Source: CAD feature listing. Evaluate the final solid. Frame: model axes, mm. Give positions to 0.01 mm unless a question says otherwise; leave off trailing zeros. Order: outer loops, then holes, each group sorted by start corner. A loop starts at its lowest first (then second) coordinate and runs counter-clockwise, first axis right, second up.
```python
from build123d import *

# Parameters (mm, degrees)
SKETCH1_R           = 88.9
SKETCH1_R_2         = 2
BOSS_EXTRUDE1_DEPTH = 1.016
SKETCH3_R           = 1.25
SKETCH3_R_2         = 2.25
CUT_EXTRUDE2_DEPTH  = 3.175
SKETCH4_R           = 4.2
CUT_EXTRUDE3_DEPTH  = 10


with BuildPart() as part:
    # Sketch1 → Boss-Extrude1 (new body)
    with BuildSketch(Plane.XY):
        Circle(SKETCH1_R)
        with Locations((41.275, 71.490397082)):
            Circle(SKETCH1_R_2, mode=Mode.SUBTRACT)
        with Locations((82.55, 0)):
            Circle(SKETCH1_R_2, mode=Mode.SUBTRACT)
        with Locations((41.275, -71.490397082)):
            Circle(SKETCH1_R_2, mode=Mode.SUBTRACT)
        with Locations((-41.275, -71.490397082)):
            Circle(SKETCH1_R_2, mode=Mode.SUBTRACT)
        with Locations((-82.55, 0)):
            Circle(SKETCH1_R_2, mode=Mode.SUBTRACT)
        with Locations((-41.275, 71.490397082)):
            Circle(SKETCH1_R_2, mode=Mode.SUBTRACT)
    extrude(amount=BOSS_EXTRUDE1_DEPTH)

    # Sketch3 → Cut-Extrude2 (cut)
    with BuildSketch(Plane.XY.offset(1.016)):
        with Locations((-46.5, 40.2)):
            Circle(SKETCH3_R)
        with Locations((46.5, 40.2)):
            Circle(SKETCH3_R)
        with Locations((46.5, -14.8)):
            Circle(SKETCH3_R)
        with Locations((-46.5, -14.8)):
            Circle(SKETCH3_R)
        with Locations((-31.700000009, 45.8)):
            Circle(SKETCH3_R_2)
    extrude(amount=-CUT_EXTRUDE2_DEPTH, mode=Mode.SUBTRACT)

    # Sketch4 → Cut-Extrude3 (cut)
    with BuildSketch(Plane.XY.offset(1.016)):
        with Locations((60.96, 29.21)):
            Circle(SKETCH4_R)
        with Locations((60.96, 13.97)):
            Circle(SKETCH4_R)
        with Locations((60.96, -1.27)):
            Circle(SKETCH4_R)
        with Locations((58.42, -21.59)):
            Circle(SKETCH4_R)
        with Locations((48.26, -36.83)):
            Circle(SKETCH4_R)
        with Locations((-58.42, -21.59)):
            Circle(SKETCH4_R)
        with Locations((-48.26, -36.83)):
            Circle(SKETCH4_R)
    extrude(amount=-CUT_EXTRUDE3_DEPTH, mode=Mode.SUBTRACT)


solid = part.part
```
1) Section query A-A, the plane y = 29.21. Return the cut outline in (x, z).
Report:
outline: (-83.96, 0) - (56.76, 0) - (56.76, 1.02) - (-83.96, 1.02) - close; (65.16, 0) - (83.96, 0) - (83.96, 1.02) - (65.16, 1.02) - close
2) Draft query along X for faces 1 (the flat face through (-1, 1, 1.016)), 2 (the cylindrical face through (-41.709, -73.443, 0.501)), 3 (the cylindrical face through (84.795, 26.703, 0.501)). Return one class per face: +X half, -X half, draft (parallel to the pull), parting line (faces both ways), or undercut.
Report:
face 1: draft
face 2: undercut
face 3: parting line
3) Section query B-B, the plane x = -58.42. Return the cut outline in (y, z), and give its area (3 significant figures).
Report:
outline: (-67.01, 0) - (-25.79, 0) - (-25.79, 1.02) - (-67.01, 1.02) - close; (-17.39, 0) - (67.01, 0) - (67.01, 1.02) - (-17.39, 1.02) - close
area: 128 mm2
4) Material intervals for L1, parallel to X at y = -71.5, z = 0.3; L2, parallel to Y at x = 60.96, z = 0.6; L3, parallel to X at y = -19.5, z = 0.85 (3 decimals), sorted ascending.
Report:
L1: x = -52.83 to -43.27, -39.28 to 39.28, 43.27 to 52.83
L2: y = -64.71 to -24.93, -18.25 to -5.47, 2.93 to 9.77, 18.17 to 25.01, 33.41 to 64.71
L3: x = -86.735 to -62.063, -54.777 to 54.777, 62.063 to 86.735
5) Section query D-D, the plane y = -21.59. Return the cut outline in (x, z).
Report:
outline: (-86.24, 0) - (-62.62, 0) - (-62.62, 1.02) - (-86.24, 1.02) - close; (-54.22, 0) - (54.22, 0) - (54.22, 1.02) - (-54.22, 1.02) - close; (62.62, 0) - (86.24, 0) - (86.24, 1.02) - (62.62, 1.02) - close
6) Section query C-C, the plane z = 0.4. Count the separate pieces of the cut face and the enclosed holes in it, and give its area (3 significant figures).
Report:
separate pieces: 1
enclosed holes: 18
area: 24,300 mm2
